```python
from build123d import *

# Parameters (mm, degrees)
SKETCH_1_R      = 10
EXTRUDE_1_DEPTH = 180
CHAMFER_1_SIZE  = 1.5
M8X1_0_1_D      = 7


with BuildPart() as part:
    # 草图1 → 凸台-拉伸1 (new body)
    with BuildSketch(Plane.XY):
        with Locations(Location((0, 0, 0), (0, 0, 180))):
            Circle(SKETCH_1_R)
    extrude(amount=EXTRUDE_1_DEPTH)

    # 倒角1
    chamfer_1_edges = [part.edges().sort_by_distance(p)[0] for p in [
        (10, 0, 0),
        (10, 0, 180),
    ]]
    chamfer(chamfer_1_edges, length=CHAMFER_1_SIZE)

    # M8x1.0 螺纹孔1 (through all)
    with Locations(Plane.XY.offset(180)):
        with Locations((0, 0)):
            Hole(M8X1_0_1_D / 2)


solid = part.part
```
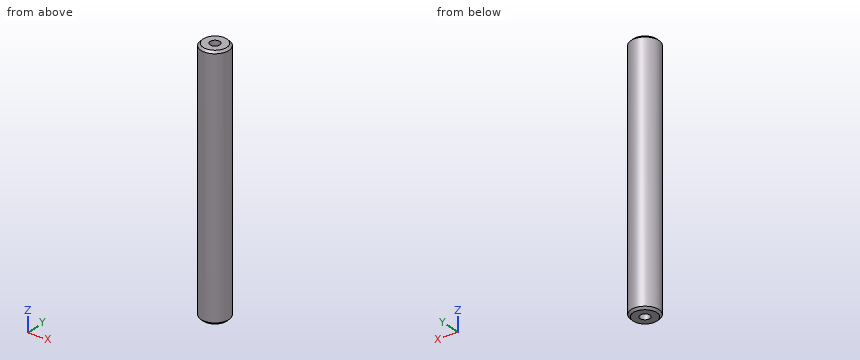
Part model, mm, in its own coordinate system. Round coordinates to 2 decimals unless told otherwise and drop trailing zeros. Order: outer loops, then holes, each group sorted by start corner. A loop starts at its lowest first (then second) coordinate and runs counter-clockwise, first axis right, second up. Notation, with made-up numbers: M -25,5 L 33,5 A23 ccw 33,35 Z; hole C -35,55.25 d5. An arc over 180 degrees is marked long. Answer in a Markdown table with one row per item. Add a question column.
Q1. Cut at A-A on x = 0. Give the cut face in (y, z).
Q2. Wall check: L1, parallel to Y at x = 0, z = 83.5; L2, parallel to Y at x = -3.75, z = 166.5; L3, parallel to X at y = -2.75, z = 120. Give the ranges that are in metal, low to high. Write a range as from..to.
Q3. Cut at C-C on z = 60. Give the cut face in (x, y).
Q4. Pin check, flat tips, straight feed: pin 1 (12 mm diameter, centred on x = 6, y = 6.5, fed in from -Z); pin 2 (5 mm diameter, centred on x = -4, z = 78.5, fed in from -Y); pin 3 (6 mm diameter, centred on x = -8, z = 63, fed in from -Y); pin 4 (3 mm diameter, centred on y = -7, z = 36, fed in from +X). Stop position of each tip, or through.
Established:
| question | item | result |
|---|---|---|
| 1 | outline | M -10,1.5 L -8.5,0 L -3.5,0 L -3.5,180 L -8.5,180 L -10,178.5 Z; M 3.5,0 L 8.5,0 L 10,1.5 L 10,178.5 L 8.5,180 L 3.5,180 Z |
| 2 | L1 | y = -10..-3.5, 3.5..10 |
| 2 | L2 | y = -9.27..9.27 |
| 2 | L3 | x = -9.61..-2.17, 2.17..9.61 |
| 3 | outline | C 0,0 d20; hole C 0,0 d7 |
| 4 | pin 1 | stops at z = 0 |
| 4 | pin 2 | stops at y = -9.89 |
| 4 | pin 3 | stops at y = -8.66 |
| 4 | pin 4 | stops at x = 8.35 |
